For this review, take the finished solid that the model builds, in its own axes (mm). Face numbers are marked on the shaded views. A direction names the side the tool comes from. Coordinates: 2 decimals unless noted, no trailing zeros. Loops run counter-clockwise (first coordinate to the right, second up) from the corner with the lowest first, then second, coordinate; pieces in that order, holes last.
1. Clearance check with flat-ended pins moving along their axes: P1, Ø3, axis at x = -14, z = -110.5, coming from the +Y side; P2, Ø18.5, axis at y = 25.5, z = -11, coming from the -X side; P3, Ø4, axis at y = 23.5, z = -117.5, coming from the +X side. State where each tip first meets the part, or that it passes through.
2. Machinability: for the marked faces 4, 5 and 6, which of the approach directions +Z, -Z, +X, -X, +Y, -Y give a long, thin tool a straight path to every point of the face, cutting with its end or side? Answer none if there is none.
3. Take a section at D-D, the plane x = 21.5. State the section outline as (y, z) points, then the cut area to 3 significant figures.
4. Mouldability with a two-part tool opening along X and no side actions: class the marked faces 1, 2 and 3 as pulls with the +X half, pulls with the -X half, needs draft (parallel to the pull), parting line crosses it, or undercut.
5. To check wall thickness, follow probe 1 along Y at (x, z) = (12.75, -12.7); probe 2 along Z at (x, y) = (15, 16); probe 3 along X at (y, z) = (18, -24). State the ranges of each line that lie inside material, in increasing order.
6. Take a section at A-A, the plane z = -12.7. State the section outline as (x, y) points.
7. Take a section at B-B, the plane y = -29. State the section outline as (x, z) points.
8. Take a section at C-C, the plane x = 0. State the section outline as (y, z) points, then the cut area to 3 significant figures.
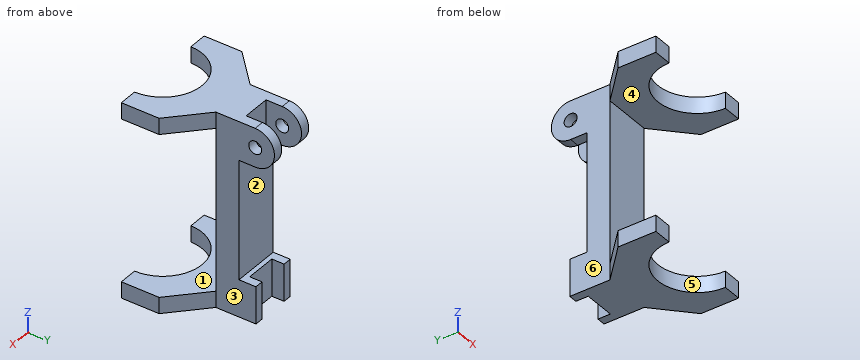
```python
from build123d import *

# Parameters (mm, degrees)
BOSS_EXTRUDE1_DEPTH = 10.16
BOSS_EXTRUDE2_START = 9.144
SKETCH1_3_R         = 4.2418
BOSS_EXTRUDE2_DEPTH = 1.016
BOSS_EXTRUDE3_START = 10.16
SKETCH1_4_R         = 4.2418
SKETCH1_4_W         = 24.384
SKETCH1_4_H         = 8.128
SKETCH1_4_H_2       = 3.048
BOSS_EXTRUDE3_DEPTH = 5.588
BOSS_EXTRUDE4_DEPTH = 10.668
BOSS_EXTRUDE6_START = -128.016
BOSS_EXTRUDE6_DEPTH = 10.668


with BuildPart() as part:
    # Sketch1 → Boss-Extrude1 (new body)
    with BuildSketch(Plane(origin=(0, 0, 0), x_dir=(0, 0, -1), z_dir=(1, 0, 0))):
        Polygon((0, 15.24), (0, 0), (128.016, 0), (128.016, 18.288), (103.632, 18.288), (103.632, 15.24), align=None)
    boss_extrude1 = extrude(amount=BOSS_EXTRUDE1_DEPTH)

    # Sketch1<3> → Boss-Extrude2 (add)
    with BuildSketch(Plane(origin=(0, 0, 0), x_dir=(0, 0, -1), z_dir=(1, 0, 0)).offset(BOSS_EXTRUDE2_START)):
        with BuildLine():
            Line((0, 25.908), (0, 15.24))
            Line((0, 15.24), (25.4, 15.24))
            Line((25.4, 15.24), (25.4, 25.908))
            ThreePointArc((25.4, 25.908), (12.7, 38.608), (0, 25.908))
        make_face()
        with Locations((12.7, 25.908)):
            Circle(SKETCH1_3_R, mode=Mode.SUBTRACT)
    boss_extrude2 = extrude(amount=BOSS_EXTRUDE2_DEPTH)

    # Sketch1<4> → Boss-Extrude3 (add)
    with BuildSketch(Plane(origin=(0, 0, 0), x_dir=(0, 0, -1), z_dir=(1, 0, 0)).offset(BOSS_EXTRUDE3_START)):
        with BuildLine():
            Line((25.4, 15.24), (25.4, 25.908))
            ThreePointArc((25.4, 25.908), (12.7, 38.608), (0, 25.908))
            Line((0, 25.908), (0, 15.24))
            Line((0, 15.24), (25.4, 15.24))
        make_face()
        with Locations((12.7, 25.908)):
            Circle(SKETCH1_4_R, mode=Mode.SUBTRACT)
        Polygon((25.4, 15.24), (128.016, 15.24), (128.016, 0), (0, 0), (0, 15.24), align=None)
        with Locations((115.824, 22.352)):
            Rectangle(SKETCH1_4_W, SKETCH1_4_H)
        with Locations((115.824, 16.764)):
            Rectangle(SKETCH1_4_W, SKETCH1_4_H_2)
    boss_extrude3 = extrude(amount=BOSS_EXTRUDE3_DEPTH)

    # Mirror3: Boss-Extrude1, Boss-Extrude2, Boss-Extrude3 across plane
    add(boss_extrude1.mirror(Plane(origin=(0, 0, 0), x_dir=(0, 0, 1), z_dir=(1, 0, 0))))
    add(boss_extrude2.mirror(Plane(origin=(0, 0, 0), x_dir=(0, 0, 1), z_dir=(1, 0, 0))))
    add(boss_extrude3.mirror(Plane(origin=(0, 0, 0), x_dir=(0, 0, 1), z_dir=(1, 0, 0))))

    # Sketch2 → Boss-Extrude4 (add)
    with BuildSketch(Plane.XY):
        with BuildLine():
            Line((25.908, -46.228), (38.1, -46.228))
            Line((38.1, -46.228), (38.1, -21.336))
            Line((38.1, -21.336), (15.748, 0))
            Line((15.748, 0), (-15.748, 0))
            Line((-15.748, 0), (-38.1, -21.336))
            Line((-38.1, -21.336), (-38.1, -46.228))
            Line((-38.1, -46.228), (-25.908, -46.228))
            ThreePointArc((-25.908, -46.228), (0, -20.32), (25.908, -46.228))
        make_face()
    extrude(amount=-BOSS_EXTRUDE4_DEPTH)

    # Sketch2<2> → Boss-Extrude6 (add)
    with BuildSketch(Plane.XY.offset(BOSS_EXTRUDE6_START)):
        with BuildLine():
            ThreePointArc((-25.908, -46.228), (0, -20.32), (25.908, -46.228))
            Line((25.908, -46.228), (38.1, -46.228))
            Line((38.1, -46.228), (38.1, -21.336))
            Line((38.1, -21.336), (15.748, 0))
            Line((15.748, 0), (-15.748, 0))
            Line((-15.748, 0), (-38.1, -21.336))
            Line((-38.1, -21.336), (-38.1, -46.228))
            Line((-38.1, -46.228), (-25.908, -46.228))
        make_face()
    extrude(amount=BOSS_EXTRUDE6_DEPTH)


solid = part.part
```
Results list:
1. P1: stops at y = 26.42
1. P2: stops at x = -15.75
1. P3: stops at x = 15.75
2. face 4: +X, -X, -Y
2. face 5: +Z, -Z, -Y
2. face 6: +Z, -Z, -X, +Y
3. outline: (-31.77, -128.02) - (-5.49, -128.02) - (-5.49, -117.35) - (-31.77, -117.35) - close; (-31.77, -10.67) - (-5.49, -10.67) - (-5.49, 0) - (-31.77, 0) - close
3. area: 561 mm2
4. face 1: needs draft
4. face 2: undercut
4. face 3: pulls with the +X half
5. probe 1: y = 0 to 21.67, 30.15 to 38.61
5. probe 2: z = -128.02 to -103.63, -25.4 to 0
5. probe 3: x = -15.75 to -9.14, 9.14 to 15.75
6. outline: (-15.75, 0) - (15.75, 0) - (15.75, 21.67) - (9.14, 21.67) - (9.14, 15.24) - (-9.14, 15.24) - (-9.14, 21.67) - (-15.75, 21.67) - close; (-15.75, 30.15) - (-9.14, 30.15) - (-9.14, 38.61) - (-15.75, 38.61) - close; (9.14, 30.15) - (15.75, 30.15) - (15.75, 38.61) - (9.14, 38.61) - close
7. outline: (-38.1, -128.02) - (-19.35, -128.02) - (-19.35, -117.35) - (-38.1, -117.35) - close; (-38.1, -10.67) - (-19.35, -10.67) - (-19.35, 0) - (-38.1, 0) - close; (19.35, -128.02) - (38.1, -128.02) - (38.1, -117.35) - (19.35, -117.35) - close; (19.35, -10.67) - (38.1, -10.67) - (38.1, 0) - (19.35, 0) - close
8. outline: (-20.32, -128.02) - (18.29, -128.02) - (18.29, -103.63) - (15.24, -103.63) - (15.24, 0) - (-20.32, 0) - (-20.32, -10.67) - (0, -10.67) - (0, -117.35) - (-20.32, -117.35) - close
8. area: 2,460 mm2
